CAD build for the part. Positions are in the model's coordinates, mm. Coordinates: 2 decimals unless noted, no trailing zeros. Loops run counter-clockwise (first coordinate to the right, second up) from the corner with the lowest first, then second, coordinate; pieces in that order, holes last. Notation, with made-up numbers: (75.25, 7.25) - (87.25, 7.25) arc R17 cw to (87.25, 18.25) - close; hole circle Ø6 at (79, 13). An arc over 180 degrees is marked (long way). Put each result on its own line as item: value.
```python
from build123d import *

# Parameters (mm, degrees)
SKETCH_1_W          = 110
SKETCH_1_H          = 80
EXTRUDE_1_DEPTH     = 3
SKETCH_2_R          = 1.5
CUT_EXTRUDE_1_DEPTH = 10
SKETCH_3_R          = 1.55
SKETCH_3_R_2        = 1.5
CUT_EXTRUDE_2_DEPTH = 10


with BuildPart() as part:
    # 草图1 → 凸台-拉伸1 (new body)
    with BuildSketch(Plane.XY):
        Rectangle(SKETCH_1_W, SKETCH_1_H)
    extrude(amount=EXTRUDE_1_DEPTH)

    # 草图2 → 切除-拉伸1 (cut)
    with BuildSketch(Plane(origin=(0, 0, 0), x_dir=(-1, 0, 0), z_dir=(0, 0, -1))):
        with Locations((-13, 20.02)):
            Circle(SKETCH_2_R)
        with Locations((-13, 35.02)):
            Circle(SKETCH_2_R)
        with Locations((15, 20.02)):
            Circle(SKETCH_2_R)
        with Locations((15, 35.02)):
            Circle(SKETCH_2_R)
    extrude(amount=-CUT_EXTRUDE_1_DEPTH, mode=Mode.SUBTRACT)

    # 草图3 → 切除-拉伸2 (cut)
    with BuildSketch(Plane(origin=(0, 0, 0), x_dir=(-1, 0, 0), z_dir=(0, 0, -1))):
        with Locations((-51, -20)):
            Circle(SKETCH_3_R)
        with Locations((-51, 25)):
            Circle(SKETCH_3_R)
        with Locations((51, -20)):
            Circle(SKETCH_3_R_2)
        with Locations((51, 25)):
            Circle(SKETCH_3_R)
    extrude(amount=-CUT_EXTRUDE_2_DEPTH, mode=Mode.SUBTRACT)


solid = part.part
```
Q1. Wall check: L1, parallel to Y at x = -51, z = 1.5; L2, parallel to X at y = 19, z = 2.55. Give the ranges that are in metal, low to high. Write a range as from..to.
Determined:
L1: -40..-21.5, -18.5..23.45, 26.55..40
L2: -55..-16.1, -13.9..11.9, 14.1..55
Q2. Slice it at B-B, the plane y = 25. Give the cut face in (x, z).
Determined:
outline: (-55, 0) - (-52.55, 0) - (-52.55, 3) - (-55, 3) - close; (-49.45, 0) - (49.45, 0) - (49.45, 3) - (-49.45, 3) - close; (52.55, 0) - (55, 0) - (55, 3) - (52.55, 3) - close
Q3. Mould opens along X. For faces 1 (the cylindrical face through (13.195, 36.507, 1.479)), 2 (the flat face through (-1, 1, 3)), 3 (the flat face through (55, -1, 1)) say: +X half, -X half, draft (parallel to the pull), parting line (faces both ways), or undercut.
Determined:
face 1: undercut
face 2: draft
face 3: +X half
Q4. Slice it at A-A, the plane x = 51. Give the cut face in (y, z).
Determined:
outline: (-40, 0) - (-21.55, 0) - (-21.55, 3) - (-40, 3) - close; (-18.45, 0) - (23.45, 0) - (23.45, 3) - (-18.45, 3) - close; (26.55, 0) - (40, 0) - (40, 3) - (26.55, 3) - close
Q5. Pin check, flat tip, straight feed: pin 1 Ø2.5 at (x, y) = (13, 35.02) entering from +Z. Stop position of the tip, or through.
Determined:
pin 1: through
